Verification items for the finished model (mm, model axes). Round coordinates to 2 decimals unless told otherwise and drop trailing zeros. Loops run counter-clockwise (first coordinate to the right, second up) from the corner with the lowest first, then second, coordinate; pieces in that order, holes last. Notation, with made-up numbers: M 18.25,-26.5 L 53.25,-26.5 A13 ccw 53.25,-15.5 Z; hole C -32,-19 d4. An arc over 180 degrees is marked long. One line per item, written item: value.
from build123d import *

# Parameters (mm, degrees)
SKETCH1_W     = 10
SKETCH1_H     = 7
CHAMFER1_SIZE = 2
CHAMFER2_SIZE = 1


with BuildPart() as part:
    # Sketch1 → Revolve2 (revolve)
    with BuildSketch(Plane.XY):
        with Locations((5, 6.5)):
            Rectangle(SKETCH1_W, SKETCH1_H)
    revolve(axis=Axis((0, 0, 0), (1, 0, 0)))

    # Chamfer1
    chamfer1_edges = [part.edges().sort_by_distance(p)[0] for p in [
        (0, -10, 0),
        (10, -10, 0),
    ]]
    chamfer(chamfer1_edges, length=CHAMFER1_SIZE)

    # Chamfer2
    chamfer2_edges = [part.edges().sort_by_distance(p)[0] for p in [
        (10, -3, 0),
    ]]
    chamfer(chamfer2_edges, length=CHAMFER2_SIZE)


solid = part.part
(1) Thickness scan on L1, parallel to Z at x = 3.5, y = 0; L2, parallel to Z at x = 5.25, y = 6; L3, parallel to Z at x = 4.5, y = -1.5. Record the ranges inside material, lowest first. Write a range as from..to.
Completed:
L1: z = -10..-3, 3..10
L2: z = -8..8
L3: z = -9.89..-2.6, 2.6..9.89
(2) Mould release check, pull along Y, two halves, no side actions. Record for faces 1 (the face through (5, -3, 0)), 2 (the face through (0, -3.4, 0.1)), 3 (the face through (0.13, -1.06, 8.06)): +Y half, -Y half, draft (parallel to the pull), parting line (faces both ways), or undercut.
Completed:
face 1: undercut
face 2: draft
face 3: parting line
(3) Sectioned sample at C-C on x = 6.25. Enter the section's corners in (y, z).
Completed:
outline: C 0,0 d20; hole C 0,0 d6
(4) Sectioned sample at D-D on x = 8.25. Enter the section's corners in (y, z).
Completed:
outline: C 0,0 d19.5; hole C 0,0 d6
(5) Sectioned sample at A-A on z = 0. Enter the section's corners in (x, y).
Completed:
outline: M 0,-8 L 2,-10 L 8,-10 L 10,-8 L 10,-4 L 9,-3 L 0,-3 Z; M 0,3 L 9,3 L 10,4 L 10,8 L 8,10 L 2,10 L 0,8 Z
